The model under review builds one solid part; all positions refer to its coordinate system, in mm. A direction names the side the tool comes from. Give positions to 0.01 mm unless a question says otherwise; leave off trailing zeros. Write each loop counter-clockwise with the first axis right and the second up, starting at its lowest first coordinate (ties: lowest second). Pieces come first, ordered by that corner, then holes.
from build123d import *

# Parameters (mm, degrees)
BASE_FLANGE2_DEPTH      = 10
BASE_FLANGE2_DEPTH_BACK = 10
TAB1_DEPTH              = 3.175
FILLET2_R               = 10
M2_5_CLEARANCE_HOLE1_D  = 2.9
FILLET1_R               = 4
M2_CLEARANCE_HOLE2_D    = 2.4
SKETCH24_R              = 4.5
CUT_EXTRUDE1_DEPTH      = 10


# Sheet-metal steps are written as plain solids
with BuildPart() as part:
    # Sketch9 → Base-Flange2 (new, two sides: drawn at the far end of the back side and taken through both)
    with BuildSketch(Plane(origin=(0, 0, 0), x_dir=(0, 0, -1), z_dir=(1, 0, 0)).offset(-BASE_FLANGE2_DEPTH_BACK)):
        with BuildLine():
            Line((-346.659099477, 27.04683438), (-331.88056775, 41.825366107))
            ThreePointArc((-331.88056775, 41.825366107), (-329.63550372, 42.755302077), (-327.390439689, 41.825366107))
            Line((-327.390439689, 41.825366107), (-311.728024486, 26.162950904))
            ThreePointArc((-311.728024486, 26.162950904), (-310.798088516, 23.917886874), (-311.728024486, 21.672822843))
            Line((-311.728024486, 21.672822843), (-326.506556213, 6.894291117))
            Line((-326.506556213, 6.894291117), (-324.261492183, 4.649227086))
            Line((-324.261492183, 4.649227086), (-309.482960456, 19.427758813))
            ThreePointArc((-309.482960456, 19.427758813), (-307.623088516, 23.917886874), (-309.482960456, 28.408014934))
            Line((-309.482960456, 28.408014934), (-325.145375659, 44.070430137))
            ThreePointArc((-325.145375659, 44.070430137), (-329.63550372, 45.930302077), (-334.12563178, 44.070430137))
            Line((-334.12563178, 44.070430137), (-348.904163507, 29.291898411))
            Line((-348.904163507, 29.291898411), (-346.659099477, 27.04683438))
        make_face()
    extrude(amount=BASE_FLANGE2_DEPTH + BASE_FLANGE2_DEPTH_BACK)

    # Sketch25 → Tab1 (add)
    with BuildSketch(Plane(origin=(0, -142.782536791, 142.782536791), x_dir=(1, 0, 0), z_dir=(0, -0.7071067811865472, 0.7071067811865479))):
        with BuildLine():
            Line((-10, 254.582575695), (10, 254.582575695))
            ThreePointArc((10, 254.582575695), (11, 250), (10, 245.417424305))
            Line((10, 245.417424305), (-10, 245.417424305))
            ThreePointArc((-10, 245.417424305), (-11, 250), (-10, 254.582575695))
        make_face()
    extrude(amount=-TAB1_DEPTH)

    # Fillet2
    fillet2_edges = [part.edges().sort_by_distance(p)[0] for p in [
        (-10, 31.876320171, 315.196329723),
        (-10, 38.35706087, 321.677070422),
        (10, 38.35706087, 321.677070422),
        (10, 31.876320171, 315.196329723),
    ]]
    fillet(fillet2_edges, radius=FILLET2_R)

    # M2.5 Clearance Hole1 (through all)
    with Locations(Plane(origin=(0, 189.098030959, 189.098030959), x_dir=(1, 0, 0), z_dir=(0, 0.7071067811865477, 0.7071067811865475))):
        with Locations((-6, -222), (6, -222)):
            Hole(M2_5_CLEARANCE_HOLE1_D / 2)

    # Fillet1
    fillet1_edges = [part.edges().sort_by_distance(p)[0] for p in [
        (-10, 28.169366396, 347.781631492),
        (10, 28.169366396, 347.781631492),
        (-10, 5.771759101, 325.384024198),
        (10, 5.771759101, 325.384024198),
    ]]
    fillet(fillet1_edges, radius=FILLET1_R)

    # M2 Clearance Hole2 (through all)
    with Locations(Plane(origin=(0, -142.782536791, 142.782536791), x_dir=(1, 0, 0), z_dir=(0, -0.7071067811865472, 0.7071067811865479))):
        with Locations((0, 258), (5.656854249, 255.656854249), (8, 250), (5.656854249, 244.343145751), (0, 242), (-5.656854249, 244.343145751), (-8, 250), (-5.656854249, 255.656854249)):
            Hole(M2_CLEARANCE_HOLE2_D / 2)

    # Sketch24 → Cut-Extrude1 (cut)
    with BuildSketch(Plane(origin=(0, -142.782536791, 142.782536791), x_dir=(1, 0, 0), z_dir=(0, -0.7071067811865472, 0.7071067811865479))):
        with Locations(Location((0, 250, 0), (0, 0, 270))):
            Circle(SKETCH24_R)
    extrude(amount=-CUT_EXTRUDE1_DEPTH, mode=Mode.SUBTRACT)


solid = part.part
1) Insertion check: pin 1 (1.5 mm diameter, centred on x = -6, z = 335.5, fed in from +Y); pin 2 (17.5 mm diameter, centred on y = 34.5, z = 338.5, fed in from -X); pin 3 (4 mm diameter, centred on x = -4, y = 14, fed in from +Z). Each pin has a flat end and moves straight along its axis. Give the tip position at first contact, or say it passes through.
2) Tool access review of faces 1 (the flat face through (-0.1, 14.4, 319)), 2 (the cylindrical face through (8.859, 29.004, 346.915)): name each direction out of +Z, -Z, +X, -X, +Y, -Y from which nothing blocks a thin tool from reaching the whole face with its end or side.
3) To check wall thickness, follow probe 1 along Y at (x, z) = (-6.5, 322.5); probe 2 along X at (y, z) = (30.5, 345.5); probe 3 along Z at (x, y) = (5.25, 41.5). State the ranges of each line that lie inside material, in increasing order.
4) The part is to be moulded in two halves that separate along Z. For faces 3 (the flat face through (-0.14, 34.333, 339.373)), 4 (the cylindrical face through (-0.14, 45.93, 329.57)), 5 (the flat face through (4.735, 36.13, 317.205)), 6 (the cylindrical face through (8.26, 34.304, 317.593)), say which applies: +Z half, -Z half, draft (parallel to the pull), parting line (faces both ways), or undercut.
5) Consider section B-B, the plane z = 318.5. State how many separate pieces and enclosed holes the cut face has, then the cut area to 3 significant figures.
6) Consider section D-D, the plane y = 25. Give the boundary of the cut face in (x, z), then the cut area to 3 significant figures.
Answer block:
1. pin 1: stops at y = 43.45
1. pin 2: stops at x = -10
1. pin 3: stops at z = 321.4
2. face 1: +Z, +X, -X
2. face 2: +Z, +X, -Y
3. probe 1: y = 6.41 to 6.62, 10.47 to 10.9, 36.93 to 37.85, 40.26 to 41.43
3. probe 2: x = -9.93 to -7.25, -4.75 to 4.75, 7.25 to 9.93
3. probe 3: z = 322.57 to 327.07, 332.21 to 336.7
4. face 3: undercut
4. face 4: parting line
4. face 5: -Z half
4. face 6: undercut
5. separate pieces: 3
5. enclosed holes: 2
5. area: 136 mm2
6. outline: (-10, 307.72) - (10, 307.72) - (10, 310.99) - (-10, 310.99) - close
6. area: 65.4 mm2
